Build history of the part. All positions in model axes, mm. A direction names the side the tool comes from. Give positions to 0.01 mm unless a question says otherwise; leave off trailing zeros. Write each loop counter-clockwise with the first axis right and the second up, starting at its lowest first coordinate (ties: lowest second). Pieces come first, ordered by that corner, then holes.
from build123d import *

# Parameters (mm, degrees)
SKETCH1_R           = 2.7
BOSS_EXTRUDE1_DEPTH = 12.7
TOP_HOLE_REACH      = 14.7
SKETCH3_R           = 2.7
SKETCH3_W           = 25.4
SKETCH3_H           = 12.7
BACK_HOLES_REACH    = 14.7
SKETCH4_R           = 2.7


with BuildPart() as part:
    # Sketch1 → Boss-Extrude1 (new body)
    with BuildSketch(Plane(origin=(0, 0, 0), x_dir=(0, -1, 0), z_dir=(-1, 0, 0))):
        Polygon((-381, 0), (-381, -116.84), (-88.9, -233.68), (0, -233.68), (0, 0), align=None)
        with Locations((-212.725, -40.64)):
            Circle(SKETCH1_R, mode=Mode.SUBTRACT)
        with Locations((-317.5, -40.64)):
            Circle(SKETCH1_R, mode=Mode.SUBTRACT)
        with Locations((-107.95, -40.64)):
            Circle(SKETCH1_R, mode=Mode.SUBTRACT)
        with Locations((-33.866666667, -193.04)):
            Circle(SKETCH1_R, mode=Mode.SUBTRACT)
        with Locations((-33.866666667, -40.64)):
            Circle(SKETCH1_R, mode=Mode.SUBTRACT)
        with Locations((-33.866666667, -116.84)):
            Circle(SKETCH1_R, mode=Mode.SUBTRACT)
    extrude(amount=-BOSS_EXTRUDE1_DEPTH)

    # Sketch3 → top hole (cut, up to next)
    with BuildSketch(Plane(origin=(12.7, 0, 0), x_dir=(0, 0, -1), z_dir=(1, 0, 0)), mode=Mode.PRIVATE) as top_hole_sk1:
        with Locations((60.96, 374.65)):
            Circle(SKETCH3_R)
    top_hole_tool1 = extrude(top_hole_sk1.sketch, amount=-TOP_HOLE_REACH, mode=Mode.PRIVATE) & part.part
    add(top_hole_tool1.solids().sort_by_distance((12.7, 374.65, -60.96))[0], mode=Mode.SUBTRACT)
    # Sketch3 → top hole (cut, up to next)
    with BuildSketch(Plane(origin=(12.7, 0, 0), x_dir=(0, 0, -1), z_dir=(1, 0, 0)), mode=Mode.PRIVATE) as top_hole_sk2:
        with Locations((12.7, 374.65)):
            Rectangle(SKETCH3_W, SKETCH3_H)
    top_hole_tool2 = extrude(top_hole_sk2.sketch, amount=-TOP_HOLE_REACH, mode=Mode.PRIVATE) & part.part
    add(top_hole_tool2.solids().sort_by_distance((12.7, 374.65, -12.7))[0], mode=Mode.SUBTRACT)
    # Sketch3 → top hole (cut, up to next)
    with BuildSketch(Plane(origin=(12.7, 0, 0), x_dir=(0, 0, -1), z_dir=(1, 0, 0)), mode=Mode.PRIVATE) as top_hole_sk3:
        with Locations((109.22, 374.65)):
            Rectangle(SKETCH3_W, SKETCH3_H)
    top_hole_tool3 = extrude(top_hole_sk3.sketch, amount=-TOP_HOLE_REACH, mode=Mode.PRIVATE) & part.part
    add(top_hole_tool3.solids().sort_by_distance((12.7, 374.65, -109.22))[0], mode=Mode.SUBTRACT)

    # Sketch4 → back holes (cut, up to next)
    with BuildSketch(Plane(origin=(12.7, 0, 0), x_dir=(0, 0, -1), z_dir=(1, 0, 0)), mode=Mode.PRIVATE) as back_holes_sk1:
        with Locations((157.754188244, 261.616631128)):
            Circle(SKETCH4_R)
    back_holes_tool1 = extrude(back_holes_sk1.sketch, amount=-BACK_HOLES_REACH, mode=Mode.PRIVATE) & part.part
    add(back_holes_tool1.solids().sort_by_distance((12.7, 261.616631, -157.754188))[0], mode=Mode.SUBTRACT)
    # Sketch4 → back holes (cut, up to next)
    with BuildSketch(Plane(origin=(12.7, 0, 0), x_dir=(0, 0, -1), z_dir=(1, 0, 0)), mode=Mode.PRIVATE) as back_holes_sk2:
        with Locations((195.487480961, 167.283399334)):
            Circle(SKETCH4_R)
    back_holes_tool2 = extrude(back_holes_sk2.sketch, amount=-BACK_HOLES_REACH, mode=Mode.PRIVATE) & part.part
    add(back_holes_tool2.solids().sort_by_distance((12.7, 167.283399, -195.487481))[0], mode=Mode.SUBTRACT)
    # Sketch4 → back holes (cut, up to next)
    with BuildSketch(Plane(origin=(12.7, 0, 0), x_dir=(0, 0, -1), z_dir=(1, 0, 0)), mode=Mode.PRIVATE) as back_holes_sk3:
        Polygon((156.575022846, 247.466646359), (184.874992385, 176.716722513), (196.666646359, 181.433384103), (168.366676821, 252.183307948), align=None)
    back_holes_tool3 = extrude(back_holes_sk3.sketch, amount=-BACK_HOLES_REACH, mode=Mode.PRIVATE) & part.part
    add(back_holes_tool3.solids().sort_by_distance((12.7, 214.450015, -176.620835))[0], mode=Mode.SUBTRACT)


solid = part.part
1. Saw through at A-A on x = 2. Count the separate pieces of the cut face and the enclosed holes in it, plus the area to 3 significant figures.
2. Drop flat-ended pins along their axis: pin 1 (3 mm diameter, centred on x = 8.5, z = -143, fed in from +Y); pin 2 (3 mm diameter, centred on y = 374.65, z = -60.96, fed in from +X); pin 3 (1.5 mm diameter, centred on x = 8, z = -112.5, fed in from +Y); pin 4 (6 mm diameter, centred on x = 6, y = 316, fed in from -Z). Give the stop position or say it passes through.
3. Mould opens along Y. For faces 5 (the face through (6, 368.3, -109)), 6 (the face through (6, 375, -25.4)), 7 (the face through (6.439, 249.858, -162.553)) say: pulls with the +Y half, pulls with the -Y half, needs draft (parallel to the pull), parting line crosses it, or undercut.
4. Drill centre lines: line 1 along Z through (x, y) = (9.75, 374.65); line 2 along Y through (x, z) = (5, -60.96); line 3 along Y through (x, z) = (10, -193.04). Where is each one in solid material? Low to high.
5. Saw through at C-C on y = 187.5. Give the cut face in (x, z).
6. 3-axis set-ups, long thin cutter, end or side, ignore diameter. For faces 1 (the face through (6.439, 179.042, -190.688)), 2 (the face through (6, 0, -118)), 3 (the face through (6, 368.3, -13)), 4 (the face through (6, 375, -96.52)): which of +Z, -Z, +X, -X, +Y, -Y reach the whole face in a straight line?
7. Saw through at B-B on y = 146.5. Give the cut face in (x, z).
Outcome:
1. separate pieces: 1
1. enclosed holes: 9
1. area: 70,200 mm2
2. pin 1: stops at y = 319.35
2. pin 2: passes through
2. pin 3: stops at y = 368.3
2. pin 4: stops at z = -144.04
3. face 5: pulls with the +Y half
3. face 6: needs draft
3. face 7: undercut
4. line 1: z = -96.52 to -63.66, -58.26 to -25.4
4. line 2: y = 0 to 371.95, 377.35 to 381
4. line 3: y = 0 to 31.17, 36.57 to 166.14, 168.42 to 179.98
5. outline: (0, -180.56) - (12.7, -180.56) - (12.7, 0) - (0, 0) - close
6. face 1: +X, -X, +Y
6. face 2: +Z, -Z, +X, -X, -Y
6. face 3: +Z, +X, -X, +Y
6. face 4: -Z, +X, -X, +Y
7. outline: (0, -210.64) - (12.7, -210.64) - (12.7, 0) - (0, 0) - close
